from build123d import *

# Parameters (mm, degrees)
F1_DEPTH = 63.5
F0_W     = 25.4
F0_H     = 19.0499988828
F2_DEPTH = 25.4
F3_DEPTH = 7.9375
F5_R     = 6.35


# Not quite as in the source:
# - ends of sketch curves that miss each other by under 0.0002 mm in the source are joined


with BuildPart() as f1:
    # F0 (on Front) → F1 (new body, symmetric)
    with BuildSketch(Plane.XZ):
        Polygon((41.275, -9.525), (41.275, 9.525), (22.2249999642, 9.525), (-41.275, 9.525), (-41.275, -9.525), align=None)
    extrude(amount=F1_DEPTH, both=True)

    # F0 (on Front) → F2 (join, symmetric)
    with BuildSketch(Plane.XZ):
        with Locations((73.025, 52.4001994414)):
            Rectangle(F0_W, F0_H)
        with BuildLine():
            Line((22.2249999642, 9.525), (41.275, 9.525))
            Line((41.275, 9.525), (41.275, 27.0002))
            ThreePointArc((41.275, 27.0002), (45.9246798487, 38.2255201513), (57.15, 42.8752))
            Line((57.15, 42.8752), (60.325, 42.8752))
            Line((60.325, 42.8752), (60.325, 61.9251988828))
            Line((60.325, 61.9251988828), (57.15, 61.9251988828))
            add(Edge.make_bspline(
                [(55.577466475, 61.8897796164), (56.107456948, 61.9056705872), (56.6317308349, 61.9174837091), (57.15, 61.9251988828)],
                knots=[109.8639655387, 109.8639655387, 109.8639655387, 109.8639655387, 111.5045361803, 111.5045361803, 111.5045361803, 111.5045361803], degree=3))
            ThreePointArc((55.577466475, 61.8897796164), (31.9044423619, 51.133526481), (22.2249999642, 27.0002))
            Line((22.2249999642, 27.0002), (22.2249999642, 9.525))
        make_face()
    extrude(amount=F2_DEPTH, both=True)

    # F0 (on Front) → F3 (join, symmetric)
    with BuildSketch(Plane.XZ):
        with BuildLine():
            Line((-41.275, 9.525), (22.2249999642, 9.525))
            Line((22.2249999642, 9.525), (22.2249999642, 27.0002))
            ThreePointArc((22.2249999642, 27.0002), (31.9044423619, 51.133526481), (55.577466475, 61.8897796164))
            add(Edge.make_bspline(
                [(-41.275, 9.525), (-41.042616605, 41.4740477998), (20.0856360221, 60.8256102231), (55.577466475, 61.8897796164)],
                knots=[0, 0, 0, 0, 109.8639655387, 109.8639655387, 109.8639655387, 109.8639655387], degree=3))
        make_face()
    extrude(amount=F3_DEPTH, both=True)

    # F0 (on Front) → F4 (revolve)
    with BuildSketch(Plane.XZ):
        Polygon((85.725, 61.9251988828), (85.725, 42.8752), (85.725, 38.1), (111.125, 38.1), (111.125, 66.675), (85.725, 66.675), align=None)
    revolve(axis=Axis((85.725, 0, 52.3875), (0, 0, 1)))

    # F5
    f5_edges = [f1.edges().sort_by_distance(p)[0] for p in [
        (41.275, -63.5, 0),
        (41.275, 63.5, 0),
        (-41.275, -63.5, 0),
        (-41.275, 63.5, 0),
    ]]
    fillet(f5_edges, radius=F5_R)


solid = f1.part
Build history of the part. All positions in model axes, mm. A direction names the side the tool comes from. Coordinates: 2 decimals unless noted, no trailing zeros. Write each loop counter-clockwise with the first axis right and the second up, starting at its lowest first coordinate (ties: lowest second). Pieces come first, ordered by that corner, then holes.
(1) Cut at A-A on z = 1. List the corners of the cut face in (x, y) (3 decimals).
(2) Cut at B-B on y = -31.5. List the corners of the cut face in (x, z) (3 decimals).
(3) Pin check, flat tips, straight feed: pin 1 Ø6 at (x, z) = (-0.5, 17.5) entering from +Y; pin 2 Ø23 at (x, y) = (66, -5.5) entering from -Z; pin 3 Ø1.5 at (x, y) = (39, -39) entering from +Z (3 decimals). Stop position of each tip, or through.
(4) Mould opens along X. For faces 5 (the flat face through (46, -25.4, 42)), 6 (the cylindrical face through (45.8, -0.4, 38.1)), 7 (the flat face through (60, 2, 42.875)), 8 (the cylindrical face through (32.16, -16.79, 51.4)) say: pulls with the +X half, pulls with the -X half, needs draft (parallel to the pull), parting line crosses it, or undercut.
(5) 3-axis set-ups, long thin cutter, end or side, ignore diameter. For faces 1 (the flat face through (86, 0, 38.1)), 2 (the flat face through (22.225, 17, 18)), 3 (the flat face through (60, -2, 61.925)), 4 (the flat face through (46, 25.4, 42)): which of +Z, -Z, +X, -X, +Y, -Y reach the whole face in a straight line?
(6) Drill centre lines: line 1 (Z direction, x = 99, y = 18) (3 decimals); line 2 (Y direction, x = 35.5, z = 41.5); line 3 (Z direction, x = 26.5, y = -42.5) (3 decimals). Where is each one in solid material? Low to high.
Working result:
1. outline: (-41.275, -57.15) arc R6.35 ccw to (-34.925, -63.5) - (34.925, -63.5) arc R6.35 ccw to (41.275, -57.15) - (41.275, 57.15) arc R6.35 ccw to (34.925, 63.5) - (-34.925, 63.5) arc R6.35 ccw to (-41.275, 57.15) - close
2. outline: (-41.275, -9.525) - (41.275, -9.525) - (41.275, 9.525) - (-41.275, 9.525) - close
3. pin 1: stops at y = 7.94
3. pin 2: stops at z = 38.1
3. pin 3: stops at z = 9.525
4. face 5: needs draft
4. face 6: undercut
4. face 7: undercut
4. face 8: pulls with the -X half
5. face 1: -Z, +X, +Y, -Y
5. face 2: +Z, -X, +Y
5. face 3: +Z, -X
5. face 4: +Z, +X, -X, +Y
6. line 1: z = 38.1 to 66.675
6. line 2: y = -25.4 to 25.4
6. line 3: z = -9.525 to 9.525
